from build123d import *

# Parameters (mm, degrees)
SKETCH1_W           = 60
SKETCH1_H           = 90
EXTRUDE1_DEPTH      = 75
EXTRUDE2_DEPTH      = 61
EXTRUDE3_DEPTH      = 76
EXTRUDE4_DEPTH      = 25
EXTRUDE4_DEPTH_BACK = 55


with BuildPart() as part:
    # Sketch1 → Extrude1 (new body)
    with BuildSketch(Plane(origin=(0, 0, 0), x_dir=(1, 0, 0), z_dir=(0, 1, 0))):
        with Locations((30, 45)):
            Rectangle(SKETCH1_W, SKETCH1_H)
    extrude(amount=EXTRUDE1_DEPTH)

    # Sketch2 → Extrude2 (cut, through all)
    with BuildSketch(Plane(origin=(60, 0, 0), x_dir=(0, 0, -1), z_dir=(1, 0, 0))):
        Polygon((60, 75), (0, 45), (0, 75), align=None)
    extrude(amount=-EXTRUDE2_DEPTH, mode=Mode.SUBTRACT)

    # Sketch3 → Extrude3 (cut, through all)
    with BuildSketch(Plane(origin=(0, 75, 0), x_dir=(1, 0, 0), z_dir=(0, 1, 0))):
        Polygon((60, 60), (15, 0), (60, 0), align=None)
    extrude(amount=-EXTRUDE3_DEPTH, mode=Mode.SUBTRACT)

    # Sketch4 → Extrude4 (add, two sides)
    with BuildSketch(Plane(origin=(60, 0, 0), x_dir=(0, 0, -1), z_dir=(1, 0, 0))) as extrude4_sk:
        Polygon((90, 0), (15, 0), (90, 35), align=None)
    extrude(amount=EXTRUDE4_DEPTH)
    extrude(extrude4_sk.sketch, amount=-EXTRUDE4_DEPTH_BACK)


solid = part.part
Work out the finished part from the listing and answer in its coordinate system (mm). A direction names the side the tool comes from. Give positions to 0.01 mm unless a question says otherwise; leave off trailing zeros. Write each loop counter-clockwise with the first axis right and the second up, starting at its lowest first coordinate (ties: lowest second). Pieces come first, ordered by that corner, then holes. Notation, with made-up numbers: M 85,-14.75 L 106,-14.75 A34 ccw 106,21.25 Z; hole C 50,20.5 d8. An arc over 180 degrees is marked long. Answer as CSV lines item,"result".
Q1. A cutting plane is placed at D-D on y = 59. Write down the section's boundary in (x, z), plus the area to 3 significant figures.
A:
outline,"M 0,-90 L 60,-90 L 60,-60 L 36,-28 L 0,-28 Z"
area,"3,340 mm²"
Q2. A cutting plane is placed at B-B on x = 77. Write down the section's boundary in (y, z).
A:
outline,"M 0,-90 L 35,-90 L 0,-15 Z"
Q3. A cutting plane is placed at A-A on y = 69.5. Write down the section's boundary in (x, z).
A:
outline,"M 0,-90 L 60,-90 L 60,-60 L 51.75,-49 L 0,-49 Z"
Q4. A tool of negligible diameter and unlimited length cuts with its end or side. For faces 1 (the flat face through (0, 37, -44)), 2 (the flat face through (62.564, 13.366, -43.642)), from which of +Z, -Z, +X, -X, +Y, -Y can it reach the whole face along a straight path? Write none if from no direction.
A:
face 1,"+Z, -Z, -X, +Y, -Y"
face 2,"+Z, +X, +Y"
Q5. Given P1, Ø1, axis at y = 27, z = -51, coming from the +X side (3 decimals); P2, Ø1, axis at x = 10.5, y = 64, coming from the +Z side; P3, Ø15, axis at y = 57.5, z = -69, coming from the +X side, each flat-ended and moving along its own axis, determine where each tip first touches the part or whether it passes through.
A:
P1,"stops at x = 53.625"
P2,"stops at z = -37"
P3,"stops at x = 60"
Q6. A cutting plane is placed at C-C on z = -7. Write down the section's boundary in (x, y), plus the area to 3 significant figures.
A:
outline,"M 0,0 L 20.25,0 L 20.25,48.5 L 0,48.5 Z"
area,"982 mm²"
Q7. Find the intervals of material crossed by probe 1 along Y at (x, z) = (35, -30); probe 2 along Y at (x, z) = (32.5, -18.5), in increasing order. Write a range as [from, to].
A:
probe 1,"y = [0, 60]"
probe 2,"y = [0, 1.63]"
